Could you check a few things on this drawing? It's one solid part, dimensions in mm from its lowest x, y, z. A direction names the side the tool comes from. Give positions to 0.01 mm unless a question says otherwise; leave off trailing zeros. Order: outer loops, then holes, each group sorted by start corner. A loop starts at its lowest first (then second) coordinate and runs counter-clockwise, first axis right, second up. Notation, with made-up numbers: (83, 18.5) - (133, 18.5) arc R30 ccw to (133, 55.5) - close; hole circle Ø8 at (2, 82.25). An arc over 180 degrees is marked (long way). Put each result on its own line as item: value.
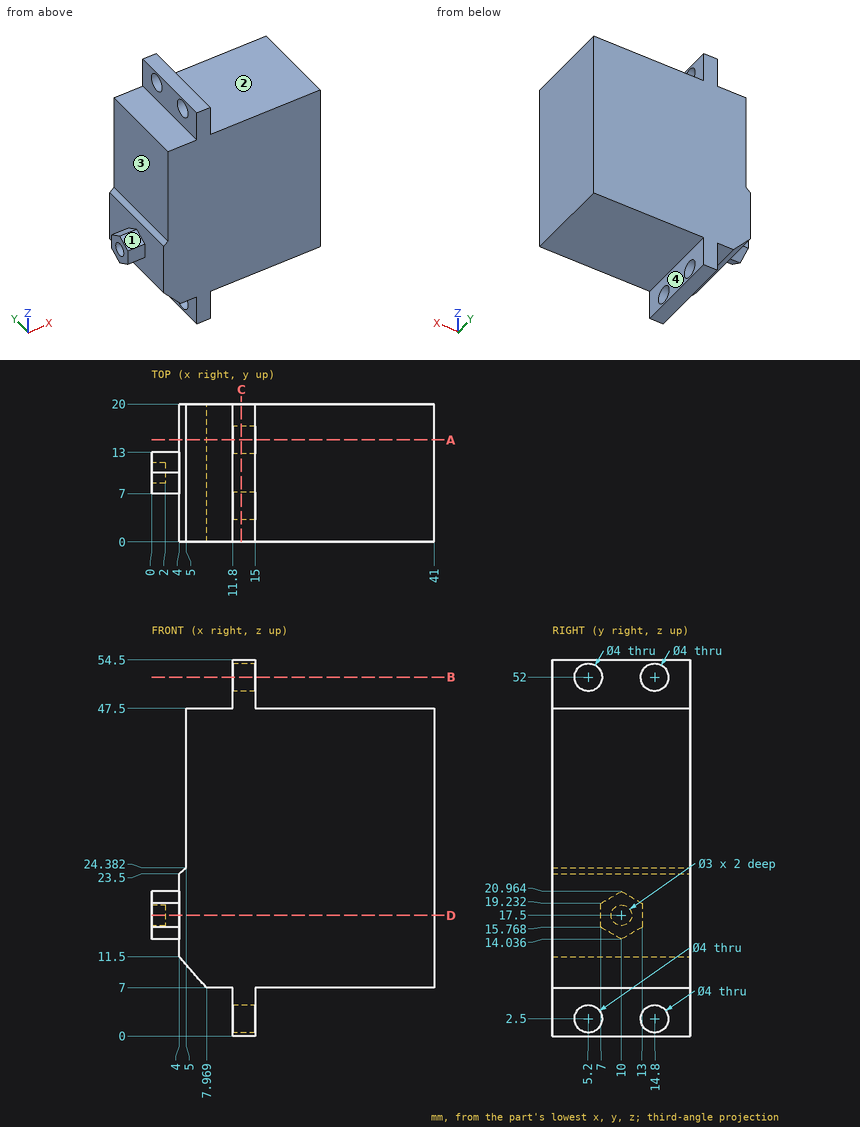
1) Which directions (+Z, -Z, +X, -X, +Y, -Y) give clear straight access to the entire face, cutting with the end or side of a thin tool? Please do the marked faces 1, 2, 3 and 4.
Filled in:
face 1: +Z, -X, -Y
face 2: +Z, +X, +Y, -Y
face 3: +Z, -X, +Y, -Y
face 4: -Z, +X, +Y, -Y
2) Suppose I cut it at B-B, the plane z = 52. List the corners of the cut face in (x, y) for me, and give its area (3 significant figures).
Filled in:
outline: (11.8, 0) - (15, 0) - (15, 3.2) - (11.8, 3.2) - close; (11.8, 7.2) - (15, 7.2) - (15, 12.8) - (11.8, 12.8) - close; (11.8, 16.8) - (15, 16.8) - (15, 20) - (11.8, 20) - close
area: 38.4 mm^2
3) Suppose I cut it at A-A, the plane y = 14.8. List the corners of the cut face in (x, z) for me.
Filled in:
outline: (4, 11.5) - (7.97, 7) - (11.8, 7) - (11.8, 4.5) - (15, 4.5) - (15, 7) - (41, 7) - (41, 47.5) - (15, 47.5) - (15, 50) - (11.8, 50) - (11.8, 47.5) - (5, 47.5) - (5, 24.38) - (4, 23.5) - close; (11.8, 0) - (15, 0) - (15, 0.5) - (11.8, 0.5) - close; (11.8, 54) - (15, 54) - (15, 54.5) - (11.8, 54.5) - close
4) If I drill on line 1 (Y direction, x = 13.8, z = 52); line 2 (Y direction, x = 0.9, z = 17.5); line 3 (Z direction, x = 10, y = 16.25), over which ranges is the centre line in solid material (lowest first)? Write a range as [from, to].
Filled in:
line 1: y = [0, 3.2], [7.2, 12.8], [16.8, 20]
line 2: y = [7, 8.5], [11.5, 13]
line 3: z = [7, 47.5]
5) Suppose I cut it at C-C, the plane x = 13. List the corners of the cut face in (y, z) for me.
Filled in:
outline: (0, 0) - (20, 0) - (20, 54.5) - (0, 54.5) - close; hole circle Ø4 at (5.2, 2.5); hole circle Ø4 at (5.2, 52); hole circle Ø4 at (14.8, 2.5); hole circle Ø4 at (14.8, 52)
6) I'm going to push flat-ended pins straight in: pin 1 (3 mm diameter, centred on x = 9.5, y = 8.5, fed in from -Z); pin 2 (5.5 mm diameter, centred on y = 7.5, z = 4, fed in from +X); pin 3 (6 mm diameter, centred on y = 6, z = 32, fed in from -X); pin 4 (3 mm diameter, centred on y = 5.2, z = 52, fed in from +X). Where does each tip first touch, or does it pass through?
Filled in:
pin 1: stops at z = 7
pin 2: stops at x = 15
pin 3: stops at x = 5
pin 4: passes through
7) Suppose I cut it at D-D, the plane z = 17.5. List the corners of the cut face in (x, y) for me, and give its area (3 significant figures).
Filled in:
outline: (0, 7) - (4, 7) - (4, 0) - (41, 0) - (41, 20) - (4, 20) - (4, 13) - (0, 13) - (0, 11.5) - (2, 11.5) - (2, 8.5) - (0, 8.5) - close
area: 758 mm^2
